For this review, take the finished solid that the model builds, in its own axes (mm). Face numbers are marked on the shaded views. A direction names the side the tool comes from. Give positions to 0.01 mm unless a question says otherwise; leave off trailing zeros. Order: outer loops, then holes, each group sorted by start corner. A loop starts at its lowest first (then second) coordinate and runs counter-clockwise, first axis right, second up. Notation, with made-up numbers: (-4, 11) -> (42, 11) arc R14 cw to (42, 36) -> close; hole circle Ø4 at (77, 44.5). An arc over 180 degrees is marked (long way). Return JSON: item names as keys, results as strings. Group by question number.
1) For the marked faces 1 and 2, list the 3-axis set-ups (+Z, -Z, +X, -X, +Y, -Y) from which the entire face can be reached by the end or side of a thin tool; tool diameter is ignored.
2) Add section A-A (y = 39.5). Give the boundary of the cut face in (x, z).
3) Add section C-C (x = 33). Give the boundary of the cut face in (y, z), then the cut area to 3 significant figures.
4) To check wall thickness, follow line 1 along X through (y, z) = (43, 7); line 2 along X through (y, z) = (32, 3.75); line 3 along Y through (x, z) = (43, 5). State the ranges of each line that lie inside material, in increasing order.
5) Add section B-B (z = 6.25). Give the boundary of the cut face in (x, y), then the cut area to 3 significant figures.
6) The part is to be moulded in two halves that separate along X. For the marked faces 3, 4 and 5, say which applies: released by +X, released by -X, zero draft, split by the parting line, or undercut.
Autodesk Inventor part; units mm, degrees
ref_plane "YZ Plane" through (0, 0, 0) normal (1, 0, 0) x (0, 1, 0)
ref_plane "XZ Plane" through (0, 0, 0) normal (0, 1, 0) x (-1, 0, 0)
ref_plane "XY Plane" through (0, 0, 0) normal (0, 0, 1) x (1, 0, 0)
sketch "Sketch1" plane through (0, 0, 0) normal (0, 0, 1) x (1, 0, 0)
  line L0 (0, 0) -> (80, 0)
  line L1 (80, 0) -> (80, 80)
  line L2 (80, 80) -> (0, 80)
  line L3 (0, 80) -> (0, 0)
  dimension "d4" = 80
  dimension "d5" = 80
extrude "Extrusion1" add sketch "Sketch1" along normal blind 10
sketch "Sketch2" plane through (0, 0, 0) normal (0, 0, -1) x (-1, 0, 0)
  line L0 (-49.5, 34.5152) -> (-49.5, 45.4848)
  line L1 (-49.5, 45.4848) -> (-40, 50.9697)
  line L2 (-40, 50.9697) -> (-30.5, 45.4848)
  line L3 (-30.5, 45.4848) -> (-30.5, 34.5152)
  line L4 (-30.5, 34.5152) -> (-40, 29.0303)
  line L5 (-40, 29.0303) -> (-49.5, 34.5152)
  point P0 (0, 0)
extrude "Extrusion2" cut sketch "Sketch2" against normal blind 20
equation "\"d4\" = 2 * nutdist"
equation "\"d5\" = 2 * nutdist"
equation "\"d0\" = nutholdert"
equation "\"d2\" = platft"
equation "\"lcsd\" = 19.05"
equation "\"lcwd1\" = 25"
equation "\"lcwd2\" = 34"
equation "\"lch1\" = 39"
equation "\"lcwd3\" = 43"
equation "\"dia1\" = 6"
equation "\"td\" = 18"
equation "\"bhh\" = 6"
equation "\"sw\" = 25"
equation "\"sh\" = 31"
equation "\"spacert\" = 2"
equation "\"platft\" = 20"
equation "\"pvct\" = 5"
equation "\"dia3\" = 8"
equation "\"dia4\" = 11"
equation "\"tankl\" = 379"
equation "\"play\" = 9"
equation "\"holeh\" = 26"
equation "\"surroundt\" = 5"
equation "\"slack\" = 0.5"
equation "\"play2\" = 3"
equation "\"diawater\" = 25"
equation "\"diaoverflow\" = 25"
equation "\"diaph\" = 32"
equation "\"diacucl\" = 32"
equation "\"diaair\" = 32"
equation "\"diasurroundhole\" = 42"
equation "\"diagrate\" = 12"
equation "\"gratespacing\" = 12.02082"
equation "\"sidedist\" = 13.9375"
equation "\"bottomdist\" = 9.6355"
equation "\"diahcl\" = 32"
equation "\"bracketwtop\" = 6"
equation "\"bracketwbottom\" = 6"
equation "\"nett\" = 1"
equation "\"nethole\" = 16"
equation "\"netside\" = 3.5"
equation "\"nettop\" = 7"
equation "\"netholespacing\" = 2"
equation "\"nutholdert\" = 10"
equation "\"diaetape\" = 32"
properties part number "platform nut holder" material "PVC-Piping"
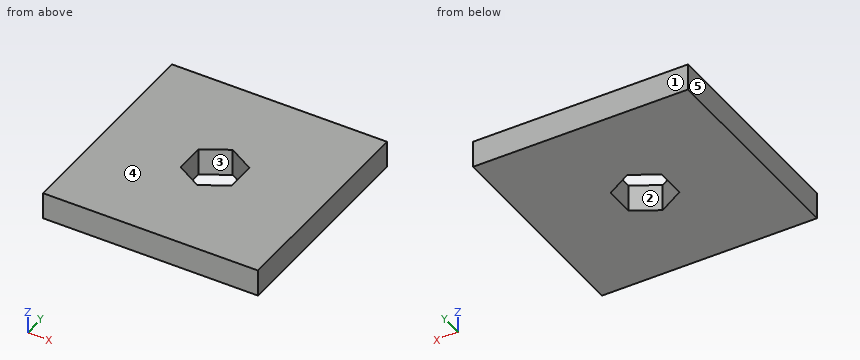
Evaluation:
{
 "1": {"face 1": "+Z, -Z, +X, -X, +Y", "face 2": "+Z, -Z"},
 "2": {"outline": "(0, 0) -> (30.5, 0) -> (30.5, 10) -> (0, 10) -> close; (49.5, 0) -> (80, 0) -> (80, 10) -> (49.5, 10) -> close"},
 "3": {"outline": "(0, 0) -> (33.07, 0) -> (33.07, 10) -> (0, 10) -> close; (46.93, 0) -> (80, 0) -> (80, 10) -> (46.93, 10) -> close", "area": "661 mm^2"},
 "4": {"line 1": "0 to 30.5, 49.5 to 80", "line 2": "0 to 34.86, 45.14 to 80", "line 3": "0 to 30.76, 49.24 to 80"},
 "5": {"outline": "(0, 0) -> (80, 0) -> (80, 80) -> (0, 80) -> close; hole (30.5, 34.52) -> (40, 29.03) -> (49.5, 34.52) -> (49.5, 45.48) -> (40, 50.97) -> (30.5, 45.48) -> close", "area": "6,090 mm^2"},
 "6": {"face 3": "undercut", "face 4": "zero draft", "face 5": "released by -X"}
}
